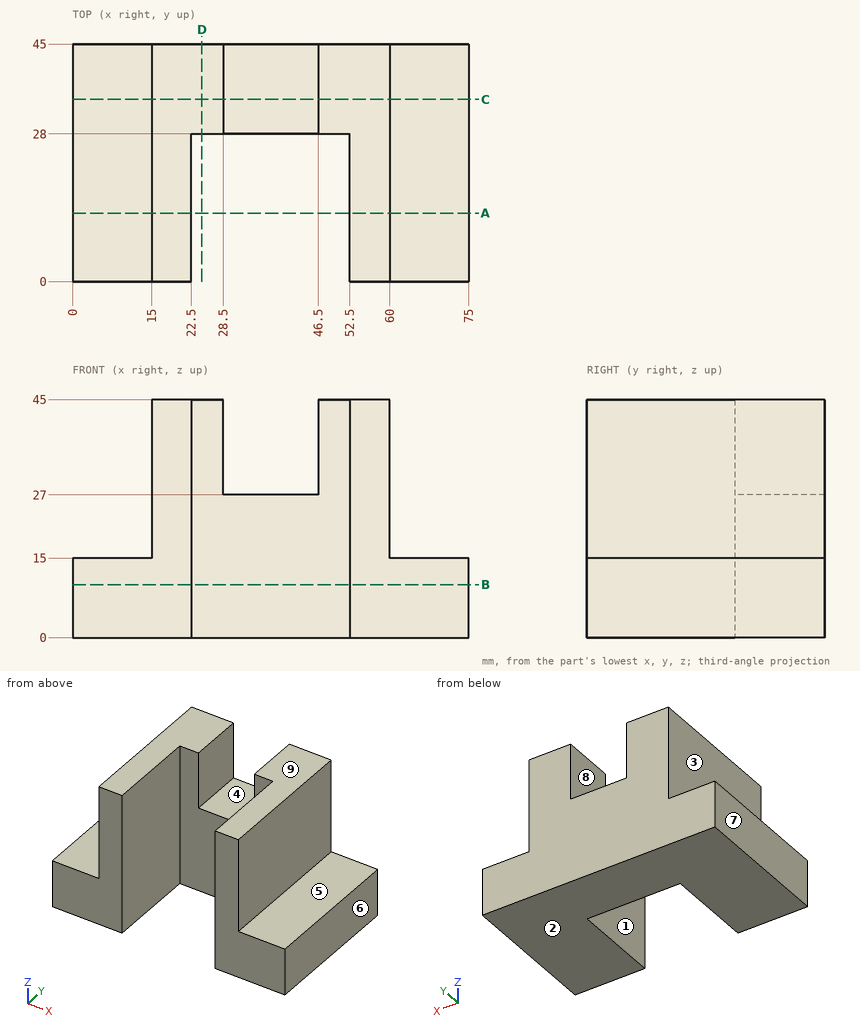
Design review of the part shown in the three views and the two pictorial views. Dimensions are in mm from the part's minimum x, y and z. A direction names the side the tool comes from. Give positions to 0.01 mm unless a question says otherwise; leave off trailing zeros. Loops run counter-clockwise (first coordinate to the right, second up) from the corner with the lowest first, then second, coordinate; pieces in that order, holes last. Notation, with made-up numbers: (42, -1) - (53, -1) arc R24 ccw to (53, 31) - close; hole circle Ø3 at (7, 32.5). An arc over 180 degrees is marked (long way). Answer as a JSON object with one key per item and string values.
Q1. Mouldability with a two-part tool opening along X and no side actions: class the marked faces 6, 7, 8 and 9 as +X half, -X half, draft (parallel to the pull), parting line (faces both ways), or undercut.
Worked out:
{"face 6": "+X half", "face 7": "-X half", "face 8": "undercut", "face 9": "draft"}
Q2. For the marked faces 1, 2, 3, 4 and 5, list the 3-axis set-ups (+Z, -Z, +X, -X, +Y, -Y) from which the entire face can be reached by the end or side of a thin tool; tool diameter is ignored.
Worked out:
{"face 1": "+Z, -Z, -Y", "face 2": "-Z, +X, -X, +Y, -Y", "face 3": "+Z, -X, +Y, -Y", "face 4": "+Z, +Y, -Y", "face 5": "+Z, +X, +Y, -Y"}
Q3. To check wall thickness, follow line 1 along X through (y, z) = (4.5, 5.5); line 2 along X through (y, z) = (39.5, 32.5); line 3 along Y through (x, z) = (38.5, 25.5). State the ranges of each line that lie inside material, in increasing order.
Worked out:
{"line 1": "x = 0 to 22.5, 52.5 to 75", "line 2": "x = 15 to 28.5, 46.5 to 60", "line 3": "y = 28 to 45"}
Q4. Insertion check: pin 1 (2 mm diameter, centred on x = 40.5, y = 40, fed in from -Z); pin 2 (12 mm diameter, centred on x = 7.5, y = 26.5, fed in from +Z); pin 3 (9 mm diameter, centred on y = 15, z = 33.5, fed in from -X); pin 4 (5 mm diameter, centred on y = 37, z = 34.5, fed in from +X). Each pin has a flat end and moves straight along its axis. Give the tip position at first contact, or say it passes through.
Worked out:
{"pin 1": "stops at z = 0", "pin 2": "stops at z = 15", "pin 3": "stops at x = 15", "pin 4": "stops at x = 60"}
Q5. Add section D-D on x = 24.5. State the section outline as (y, z) points, plus the area to 3 significant figures.
Worked out:
{"outline": "(28, 0) - (45, 0) - (45, 45) - (28, 45) - close", "area": "765 mm^2"}
Q6. Add section C-C on y = 34.5. State the section outline as (x, z) points.
Worked out:
{"outline": "(0, 0) - (75, 0) - (75, 15) - (60, 15) - (60, 45) - (46.5, 45) - (46.5, 27) - (28.5, 27) - (28.5, 45) - (15, 45) - (15, 15) - (0, 15) - close"}
Q7. Add section A-A on y = 13. State the section outline as (x, z) points, plus the area to 4 significant figures.
Worked out:
{"outline": "(0, 0) - (22.5, 0) - (22.5, 45) - (15, 45) - (15, 15) - (0, 15) - close; (52.5, 0) - (75, 0) - (75, 15) - (60, 15) - (60, 45) - (52.5, 45) - close", "area": "1,125 mm^2"}
Q8. Add section B-B on z = 10. State the section outline as (x, y) points, plus the area to 4 significant figures.
Worked out:
{"outline": "(0, 0) - (22.5, 0) - (22.5, 28) - (52.5, 28) - (52.5, 0) - (75, 0) - (75, 45) - (0, 45) - close", "area": "2,535 mm^2"}
